For this review, use the dimensioned drawing (mm, ordinates from the lowest corner) and the shaded views. Give positions to 0.01 mm unless a question says otherwise; leave off trailing zeros. Write each loop counter-clockwise with the first axis right and the second up, starting at its lowest first coordinate (ties: lowest second). Pieces come first, ordered by that corner, then holes. Notation, with made-up numbers: (15, 20.5) -> (25, 20.5) arc R10 ccw to (25, 37.5) -> close; hole circle Ø6 at (-11, 76). An arc over 180 degrees is marked (long way). Return JSON: item names as keys, results as strings.
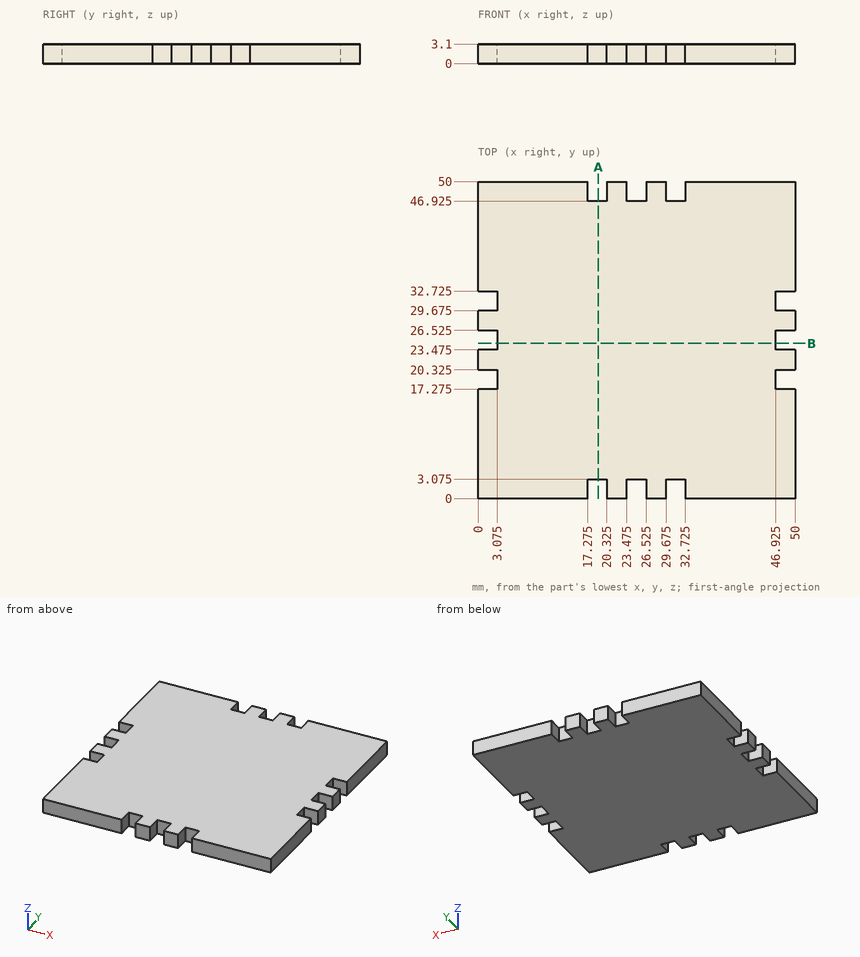
1. For pin 1 (0.9 mm diameter, centred on y = 18.5, z = 2, fed in from -X) (3 decimals); pin 2 (1.5 mm diameter, centred on x = 31.5, z = 1, fed in from +Y) (3 decimals), all flat-tipped, find the tip position at first contact; note any pin that passes through.
Results found:
{"pin 1": "stops at x = 3.075", "pin 2": "stops at y = 46.925"}
2. To check wall thickness, follow probe 1 along X at (y, z) = (3, 0.7) (3 decimals); probe 2 along Y at (x, z) = (25.5, 1.4) (3 decimals). State the ranges of each line that lie inside material, in increasing order.
Results found:
{"probe 1": "x = 0 to 17.275, 20.325 to 23.475, 26.525 to 29.675, 32.725 to 50", "probe 2": "y = 3.075 to 46.925"}
3. Add section A-A, the plane x = 19. State the section outline as (y, z) points (3 decimals).
Results found:
{"outline": "(3.075, 0) -> (46.925, 0) -> (46.925, 3.1) -> (3.075, 3.1) -> close"}
